from build123d import *

# Parameters (mm, degrees)
SKETCH_1_W           = 270
SKETCH_1_H           = 370
SKETCH_1_W_2         = 250
SKETCH_1_H_2         = 350
EXTRUDE_2_DEPTH      = 45
SKETCH_4_W           = 250
SKETCH_4_H           = 350
SKETCH_4_W_2         = 222
SKETCH_4_H_2         = 322
EXTRUDE_3_DEPTH      = 5
SKETCH_9_W           = 246
SKETCH_9_H           = 346
SKETCH_9_W_2         = 226
SKETCH_9_H_2         = 326
CUT_EXTRUDE_3_DEPTH  = 2.5
SKETCH_12_R          = 1.6
CUT_EXTRUDE_5_DEPTH  = 109.5
FILLET_1_R           = 5
SKETCH_13_W          = 250
SKETCH_13_H          = 350
SKETCH_13_W_2        = 222
SKETCH_13_H_2        = 322
EXTRUDE_4_DEPTH      = 33.5
CUT_EXTRUDE_START    = -126.5
SKETCH_14_R          = 1.6
CUT_EXTRUDE_8_DEPTH  = 126.5
SKETCH_15_W          = 209.875644348
SKETCH_15_H          = 2
CUT_EXTRUDE_9_DEPTH  = 2.5
CUT_EXTRUDE_10_DEPTH = 60.5
SKETCH_18_R          = 1.6
CUT_EXTRUDE_11_DEPTH = 60.5
SKETCH_19_W          = 30
SKETCH_19_H          = 6
CUT_EXTRUDE_12_DEPTH = 30
CUT_EXTRUDE_13_DEPTH = 30
CUT_EXTRUDE_14_DEPTH = 55


with BuildPart() as part:
    # 草图1 → 凸台-拉伸2 (new body)
    with BuildSketch(Plane(origin=(0, 0, 0), x_dir=(1, 0, 0), z_dir=(0, 1, 0))):
        with Locations((125, 175)):
            Rectangle(SKETCH_1_W, SKETCH_1_H)
        with Locations((125, 175)):
            Rectangle(SKETCH_1_W_2, SKETCH_1_H_2, mode=Mode.SUBTRACT)
    extrude(amount=EXTRUDE_2_DEPTH)

    # 草图4 → 凸台-拉伸3 (add)
    with BuildSketch(Plane(origin=(0, 38.5, 0), x_dir=(1, 0, 0), z_dir=(0, 1, 0))):
        with Locations((125, 175)):
            Rectangle(SKETCH_4_W, SKETCH_4_H)
        with Locations((125, 175)):
            Rectangle(SKETCH_4_W_2, SKETCH_4_H_2, mode=Mode.SUBTRACT)
    extrude(amount=-EXTRUDE_3_DEPTH)

    # 草图9 → 切除-拉伸3 (cut)
    with BuildSketch(Plane(origin=(0, 38.5, 0), x_dir=(1, 0, 0), z_dir=(0, 1, 0))):
        with Locations((125, 175)):
            Rectangle(SKETCH_9_W, SKETCH_9_H)
        with Locations((125, 175)):
            Rectangle(SKETCH_9_W_2, SKETCH_9_H_2, mode=Mode.SUBTRACT)
    extrude(amount=-CUT_EXTRUDE_3_DEPTH, mode=Mode.SUBTRACT)

    # 草图12 → 切除-拉伸5 (cut)
    with BuildSketch(Plane(origin=(0, 45, 0), x_dir=(1, 0, 0), z_dir=(0, 1, 0))):
        with Locations(Location((-5, -5, 0), (0, 0, 270))):
            Circle(SKETCH_12_R)
        with BuildLine():
            ThreePointArc((-6.13137085, 356.13137085), (-6.13137085, 353.86862915), (-3.86862915, 353.86862915))
            Line((-3.86862915, 353.86862915), (-6.13137085, 356.13137085))
        make_face()
        with BuildLine():
            Line((-6.13137085, 356.13137085), (-3.86862915, 353.86862915))
            ThreePointArc((-3.86862915, 353.86862915), (-3.521792748, 354.387706508), (-3.4, 355))
            ThreePointArc((-3.4, 355), (-4.387706508, 356.478207252), (-6.13137085, 356.13137085))
        make_face()
        with Locations(Location((255, 355, 0), (0, 0, 270))):
            Circle(SKETCH_12_R)
        with Locations(Location((255, -5, 0), (0, 0, 270))):
            Circle(SKETCH_12_R)
    extrude(amount=-CUT_EXTRUDE_5_DEPTH, mode=Mode.SUBTRACT)

    # 圆角1
    fillet_1_edges = [part.edges().sort_by_distance(p)[0] for p in [
        (-10, 22.5, 10),
        (-10, 22.5, -360),
        (260, 22.5, -360),
        (260, 22.5, 10),
    ]]
    fillet(fillet_1_edges, radius=FILLET_1_R)

    # 草图13 → 凸台-拉伸4 (add)
    with BuildSketch(Plane.XZ.offset(-33.5)):
        with Locations((125, -175)):
            Rectangle(SKETCH_13_W, SKETCH_13_H)
        with Locations((125, -175)):
            Rectangle(SKETCH_13_W_2, SKETCH_13_H_2, mode=Mode.SUBTRACT)
    extrude(amount=EXTRUDE_4_DEPTH)

    # 草图14 → 切除-拉伸8 (cut)
    # profile 1 of 7: a face of its own
    with BuildSketch(Plane.XZ.offset(CUT_EXTRUDE_START)):
        with BuildLine():
            Line((14, -336), (14, -14))
            Line((14, -14), (14, -6))
            Line((14, -6), (14, 2))
            Line((14, 2), (14, 10))
            Line((14, 10), (-5, 10))
            ThreePointArc((-5, 10), (-8.535533906, 8.535533906), (-10, 5))
            Line((-10, 5), (-10, -355))
            ThreePointArc((-10, -355), (-8.535533906, -358.535533906), (-5, -360))
            Line((-5, -360), (255, -360))
            ThreePointArc((255, -360), (258.535533906, -358.535533906), (260, -355))
            Line((260, -355), (260, 5))
            ThreePointArc((260, 5), (258.535533906, 8.535533906), (255, 10))
            Line((255, 10), (236, 10))
            Line((236, 10), (236, 2))
            Line((236, 2), (236, -6))
            Line((236, -6), (236, -14))
            Line((236, -14), (236, -336))
            Line((236, -336), (14, -336))
        make_face()
        with Locations((-5, -355)):
            Circle(SKETCH_14_R, mode=Mode.SUBTRACT)
        with Locations((255, -355)):
            Circle(SKETCH_14_R, mode=Mode.SUBTRACT)
        with Locations((-5, 5)):
            Circle(SKETCH_14_R, mode=Mode.SUBTRACT)
        with Locations((255, 5)):
            Circle(SKETCH_14_R, mode=Mode.SUBTRACT)
    # profile 2 of 7: a face of its own
    with BuildSketch(Plane.XZ.offset(CUT_EXTRUDE_START)):
        Polygon((14, 2), (14, -6), (20.062177826, -9.5), (20.062177826, 5.5), align=None)
    # profile 3 of 7: a face of its own
    with BuildSketch(Plane.XZ.offset(CUT_EXTRUDE_START)):
        with Locations((-5, 5)):
            Circle(SKETCH_14_R)
    # profile 4 of 7: a face of its own
    with BuildSketch(Plane.XZ.offset(CUT_EXTRUDE_START)):
        Polygon((229.937822174, -9.5), (236, -6), (236, 2), (229.937822174, 5.5), align=None)
    # profile 5 of 7: a face of its own
    with BuildSketch(Plane.XZ.offset(CUT_EXTRUDE_START)):
        with Locations((255, 5)):
            Circle(SKETCH_14_R)
    # profile 6 of 7: a face of its own
    with BuildSketch(Plane.XZ.offset(CUT_EXTRUDE_START)):
        with Locations((255, -355)):
            Circle(SKETCH_14_R)
    # profile 7 of 7: a face of its own
    with BuildSketch(Plane.XZ.offset(CUT_EXTRUDE_START)):
        with Locations((-5, -355)):
            Circle(SKETCH_14_R)
    extrude(amount=CUT_EXTRUDE_8_DEPTH, mode=Mode.SUBTRACT)

    # 草图15 → 切除-拉伸9 (cut)
    with BuildSketch(Plane(origin=(0, 38.5, 0), x_dir=(1, 0, 0), z_dir=(0, 1, 0))):
        with Locations((125, 1)):
            Rectangle(SKETCH_15_W, SKETCH_15_H)
    extrude(amount=-CUT_EXTRUDE_9_DEPTH, mode=Mode.SUBTRACT)

    # 草图16 → 切除-拉伸10 (cut)
    with BuildSketch(Plane(origin=(0, 45, 0), x_dir=(1, 0, 0), z_dir=(0, 1, 0))):
        Polygon((236, -10), (236, -8), (234, -8), (229.607695155, -8), (14, -8), (14, -10), align=None)
    extrude(amount=-CUT_EXTRUDE_10_DEPTH, mode=Mode.SUBTRACT)

    # 草图18 → 切除-拉伸11 (cut)
    with BuildSketch(Plane(origin=(0, 45, 0), x_dir=(1, 0, 0), z_dir=(0, 1, 0))):
        with Locations(Location((166, -4, 0), (0, 0, 270))):
            Circle(SKETCH_18_R)
        with Locations(Location((84, -4, 0), (0, 0, 270))):
            Circle(SKETCH_18_R)
    extrude(amount=-CUT_EXTRUDE_11_DEPTH, mode=Mode.SUBTRACT)

    # 草图19 → 切除-拉伸12 (cut)
    with BuildSketch(Plane.XZ):
        with Locations((191, -11)):
            Rectangle(SKETCH_19_W, SKETCH_19_H)
    extrude(amount=-CUT_EXTRUDE_12_DEPTH, mode=Mode.SUBTRACT)

    # 草图20 → 切除-拉伸13 (cut)
    with BuildSketch(Plane(origin=(0, 0, -8), x_dir=(-1, 0, 0), z_dir=(0, 0, -1))):
        with BuildLine():
            Line((-198.5, 26.5), (-198.5, 19))
            Line((-198.5, 19), (-195.5, 19))
            Line((-195.5, 19), (-195.5, 26.5))
            ThreePointArc((-195.5, 26.5), (-197, 28), (-198.5, 26.5))
        make_face()
        with BuildLine():
            Line((-195.5, 19), (-198.5, 19))
            Line((-198.5, 19), (-198.5, 11.5))
            ThreePointArc((-198.5, 11.5), (-197, 10), (-195.5, 11.5))
            Line((-195.5, 11.5), (-195.5, 19))
        make_face()
        with BuildLine():
            Line((-191, 10), (-191, 19))
            Line((-191, 19), (-192.5, 19))
            Line((-192.5, 19), (-192.5, 11.5))
            ThreePointArc((-192.5, 11.5), (-192.060660172, 10.439339828), (-191, 10))
        make_face()
        with BuildLine():
            Line((-189.5, 19), (-191, 19))
            Line((-191, 19), (-191, 10))
            ThreePointArc((-191, 10), (-189.939339828, 10.439339828), (-189.5, 11.5))
            Line((-189.5, 11.5), (-189.5, 19))
        make_face()
        with BuildLine():
            ThreePointArc((-189.5, 26.5), (-189.939339828, 27.560660172), (-191, 28))
            Line((-191, 28), (-191, 19))
            Line((-191, 19), (-189.5, 19))
            Line((-189.5, 19), (-189.5, 26.5))
        make_face()
        with BuildLine():
            Line((-191, 19), (-191, 28))
            ThreePointArc((-191, 28), (-192.060660172, 27.560660172), (-192.5, 26.5))
            Line((-192.5, 26.5), (-192.5, 19))
            Line((-192.5, 19), (-191, 19))
        make_face()
        with BuildLine():
            Line((-186.5, 19), (-183.5, 19))
            Line((-183.5, 19), (-183.5, 26.5))
            ThreePointArc((-183.5, 26.5), (-185, 28), (-186.5, 26.5))
            Line((-186.5, 26.5), (-186.5, 19))
        make_face()
        with BuildLine():
            Line((-183.5, 11.5), (-183.5, 19))
            Line((-183.5, 19), (-186.5, 19))
            Line((-186.5, 19), (-186.5, 11.5))
            ThreePointArc((-186.5, 11.5), (-185, 10), (-183.5, 11.5))
        make_face()
    extrude(amount=-CUT_EXTRUDE_13_DEPTH, mode=Mode.SUBTRACT)

    # 草图22 → 切除-拉伸14 (cut)
    with BuildSketch(Plane(origin=(0, 45, 0), x_dir=(1, 0, 0), z_dir=(0, 1, 0))):
        with BuildLine():
            ThreePointArc((126.6, -4), (126.13137085, -2.86862915), (125, -2.4))
            Line((125, -2.4), (125, -5.6))
            ThreePointArc((125, -5.6), (126.13137085, -5.13137085), (126.6, -4))
        make_face()
        with BuildLine():
            Line((125, -5.6), (125, -2.4))
            ThreePointArc((125, -2.4), (123.4, -4), (125, -5.6))
        make_face()
    extrude(amount=-CUT_EXTRUDE_14_DEPTH, mode=Mode.SUBTRACT)


solid = part.part
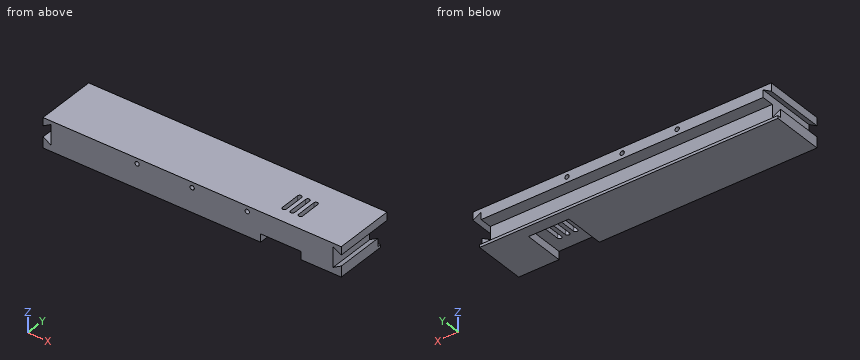
Verification items for the finished model (mm, model axes). Coordinates: 2 decimals unless noted, no trailing zeros. Order: outer loops, then holes, each group sorted by start corner. A loop starts at its lowest first (then second) coordinate and runs counter-clockwise, first axis right, second up.
1. Go/stop test with flat-tipped pins: pin 1 Ø9 at (x, y) = (197.5, 12.5) entering from -Z; pin 2 Ø4.5 at (y, z) = (17, -2) entering from +X; pin 3 Ø3.5 at (x, z) = (96.5, -7.5) entering from +Y. Record where each tip stops, or that it passes through.
Results found:
pin 1: stops at z = -8
pin 2: stops at x = 229.94
pin 3: stops at y = 36
2. Sectioned sample at C-C, the plane x = 201.5. Record the cut outline in (y, z).
Results found:
outline: (0, -8) - (30, -8) - (30, -14) - (38.5, -14) - (38.5, -12) - (36, -12) - (36, 0) - (45, 0) - (45, 8) - (0, 8) - close
3. Sectioned sample at A-A, the plane y = 16. Give the number of separate pieces and of enclosed holes in the cut face, and give its area (3 significant figures).
Results found:
separate pieces: 4
enclosed holes: 3
area: 4,400 mm2
4. Sectioned sample at D-D, the plane y = 33. Record the cut outline in (x, z), and give its area (3 significant figures).
Results found:
outline: (14, -14) - (236, -14) - (236, -6) - (229.94, -9.5) - (229.94, 5.5) - (236, 2) - (236, 8) - (14, 8) - (14, 2) - (20.06, 5.5) - (20.06, -9.5) - (14, -6) - close; hole circle Ø3.2 at (84, 4); hole circle Ø3.2 at (125, 4); hole circle Ø3.2 at (166, 4)
area: 4,720 mm2
5. Scan lines: line 1 (Z direction, x = 166, y = 11); line 2 (X direction, y = 23, z = -4.5); line 3 (X direction, y = 3, z = -11.5). Record each from-to range of solid material in increasing order.
Results found:
line 1: z = -14 to 2.4, 5.6 to 8
line 2: x = 20.06 to 183.5, 186.5 to 189.5, 192.5 to 195.5, 198.5 to 229.94
line 3: x = 14 to 176, 206 to 236
6. Sectioned sample at B-B, the plane y = 7. Record the cut outline in (x, z), and give its area (3 significant figures).
Results found:
outline: (14, -14) - (176, -14) - (176, -8) - (206, -8) - (206, -14) - (236, -14) - (236, -6) - (229.94, -9.5) - (229.94, 5.5) - (236, 2) - (236, 8) - (14, 8) - (14, 2) - (20.06, 5.5) - (20.06, -9.5) - (14, -6) - close; hole circle Ø3.2 at (84, 4); hole circle Ø3.2 at (125, 4); hole circle Ø3.2 at (166, 4)
area: 4,540 mm2
